Input: part model. Units: mm. Frame: model coordinates. A direction names the side the tool comes from. Give positions to 0.01 mm unless a question says otherwise; leave off trailing zeros. Loops run counter-clockwise (first coordinate to the right, second up) from the corner with the lowest first, then second, coordinate; pieces in that order, holes last. Notation, with made-up numbers: (68.5, 16.25) - (108.5, 16.25) arc R11 cw to (108.5, 30.25) - close; hole circle Ø11 at (58, 25). An arc over 180 degrees is marked (long way). Answer as a JSON object with one key per item and string values. Group by question number.
(1) Pin query (flat end, axial travel): P1, Ø4, axis at x = -78.5, y = 43.5, coming from the -Z side; P2, Ø10, axis at x = -23.5, y = 35, coming from the -Z side; P3, Ø6, axis at x = -40.5, y = 5, coming from the -Z side. Return the tip coordinate at first contact, or that it passes through.
(2) Mould query, pull axis X, two halves, no side actions, for faces 4 (the flat face through (-78, 43, -15.147)), 5 (the flat face through (-80, 3, 1)), 6 (the flat face through (80, 3, 1)), 7 (the flat face through (75, -4, 6)). Classes: +X half, -X half, draft (parallel to the pull), parting line (faces both ways), or undercut.
(3) Access query for faces 1 (the flat face through (77, 43, -15.147)), 2 (the flat face through (-1, -35, 6)), 3 (the flat face through (1, 37, -15.147)). Directions: +Z, -Z, +X, -X, +Y, -Y. A direction counts if a zero-diameter tool reaches every point of the face in a straight line with its end or side. Return the directions, or none.
(4) Section query C-C (y = -12.5). Return loops of the section in (x, z), plus the area to 3 significant figures.
(5) Section query A-A (z = -2). Return loops of the section in (x, y), plus the area to 3 significant figures.
(6) Section query D-D (x = 22). Return loops of the section in (y, z), plus the area to 3 significant figures.
(7) Material intervals for L1, parallel to X at y = 15, z = -1.5; L2, parallel to Y at x = 52, z = 79.5; L3, parallel to Y at x = 17.5, z = -56, sorted ascending.
(8) Section query B-B (z = -60). Return loops of the section in (x, y), plus the area to 3 significant figures.
```python
from build123d import *

# Parameters (mm, degrees)
SKETCH1_W           = 200
SKETCH1_H           = 80
BOSS_EXTRUDE1_DEPTH = 80
SKETCH2_W           = 150
SKETCH2_H           = 70
CUT_EXTRUDE2_DEPTH  = 190
FILLET5_R           = 85
CUT_EXTRUDE6_DEPTH  = 10
SKETCH9_W           = 5
SKETCH9_H           = 115.147186258
BOSS_EXTRUDE2_DEPTH = 7
SKETCH10_W          = 5
SKETCH10_H          = 115.147186258
BOSS_EXTRUDE3_DEPTH = 7
SKETCH13_W          = 100
SKETCH13_H          = 3.5
CUT_EXTRUDE9_DEPTH  = 1
SKETCH14_W          = 100
SKETCH14_H          = 3.5
CUT_EXTRUDE10_DEPTH = 1


with BuildPart() as part:
    # Sketch1 → Boss-Extrude1 (new, symmetric)
    with BuildSketch(Plane(origin=(0, 0, 0), x_dir=(0, 0, -1), z_dir=(1, 0, 0))):
        Rectangle(SKETCH1_W, SKETCH1_H)
    extrude(amount=BOSS_EXTRUDE1_DEPTH, both=True)

    # Sketch2 → Cut-Extrude2 (cut)
    with BuildSketch(Plane.XY.offset(100)):
        Rectangle(SKETCH2_W, SKETCH2_H)
    extrude(amount=-CUT_EXTRUDE2_DEPTH, mode=Mode.SUBTRACT)

    # Fillet5
    # the kernel refuses this fillet: 85 mm, written as the material it adds along each edge
    with BuildSketch(Plane(origin=(-75, 35, -90), x_dir=(0, 0, 1), z_dir=(1, 0, 0))) as fillet5_piece_1:
        with BuildLine():
            CenterArc((83.666002653, 85), FILLET5_R, 190.164248622, 79.835751378)
            Line((0, 70), (-1.673320053, 69.7))
            ThreePointArc((-1.673320053, 69.7), (-1.7, 35), (-1.7, 0))
            Line((-1.7, 0), (0, -1.7))
            Line((0, -1.7), (83.666002653, -1.7))
            Line((83.666002653, -1.7), (83.666002653, 0))
        make_face()
    extrude(amount=150)
    # the kernel refuses this fillet: 85 mm, written as the material it takes off along each edge
    with BuildSketch(Plane(origin=(-292.132034356, 40, -100), x_dir=(0, -1, 0), z_dir=(1, 0, 0))) as fillet5_2_piece_1:
        with BuildLine():
            CenterArc((85, -84.852813742), FILLET5_R, 93.372286683, 86.627713317)
            Line((0, -84.852813742), (-1.7, -84.852813742))
            Line((-1.7, -84.852813742), (-1.7, 0))
            Line((-1.7, 0), (0, 1.7))
            ThreePointArc((0, 1.7), (40, 1.7), (79.9, 1.697056275))
            Line((79.9, 1.697056275), (80, 0))
        make_face()
    extrude(amount=584.264068712, mode=Mode.SUBTRACT)

    # Sketch8 → Cut-Extrude6 (cut)
    with BuildSketch(Plane(origin=(0, 40, 0), x_dir=(1, 0, 0), z_dir=(0, 1, 0))):
        Polygon((0, 15.147186258), (-75, 15.147186258), (-75, -100), (75, -100), (75, 15.147186258), align=None)
    extrude(amount=-CUT_EXTRUDE6_DEPTH, mode=Mode.SUBTRACT)

    # Sketch9 → Boss-Extrude2 (add)
    with BuildSketch(Plane(origin=(0, 40, 0), x_dir=(1, 0, 0), z_dir=(0, 1, 0))):
        with Locations((-77.5, -42.426406871)):
            Rectangle(SKETCH9_W, SKETCH9_H)
    extrude(amount=BOSS_EXTRUDE2_DEPTH)

    # Sketch10 → Boss-Extrude3 (add)
    with BuildSketch(Plane(origin=(0, 40, 0), x_dir=(1, 0, 0), z_dir=(0, 1, 0))):
        with Locations((77.5, -42.426406871)):
            Rectangle(SKETCH10_W, SKETCH10_H)
    extrude(amount=BOSS_EXTRUDE3_DEPTH)

    # Sketch13 → Cut-Extrude9 (cut)
    with BuildSketch(Plane(origin=(-75, 0, 0), x_dir=(0, 0, -1), z_dir=(1, 0, 0))):
        with Locations((-34.852813742, 41.75)):
            Rectangle(SKETCH13_W, SKETCH13_H)
    extrude(amount=-CUT_EXTRUDE9_DEPTH, mode=Mode.SUBTRACT)

    # Sketch14 → Cut-Extrude10 (cut)
    with BuildSketch(Plane.ZY.offset(-75)):
        with Locations((34.852813742, 41.75)):
            Rectangle(SKETCH14_W, SKETCH14_H)
    extrude(amount=-CUT_EXTRUDE10_DEPTH, mode=Mode.SUBTRACT)


solid = part.part
```
Recorded:
{
 "1": {"P1": "stops at z = -15.15", "P2": "stops at z = -55.15", "P3": "stops at z = -85.97"},
 "2": {"face 4": "draft", "face 5": "-X half", "face 6": "+X half", "face 7": "undercut"},
 "3": {"face 1": "-Z, +X, -X, +Y", "face 2": "+Z", "face 3": "+Z, +Y"},
 "4": {"outline": "(-80, -93.69) - (80, -93.69) - (80, 100) - (75, 100) - (75, -82.61) - (-75, -82.61) - (-75, 100) - (-80, 100) - close", "area": "3,600 mm^2"},
 "5": {"outline": "(-80, -40) - (80, -40) - (80, 47) - (75, 47) - (75, 43.5) - (76, 43.5) - (76, 40) - (75, 40) - (75, -35) - (-75, -35) - (-75, 40) - (-76, 40) - (-76, 43.5) - (-75, 43.5) - (-75, 47) - (-80, 47) - close", "area": "1,610 mm^2"},
 "6": {"outline": "(-40, -100) arc R85 ccw to (40, -15.15) - (34.54, -15.15) arc R85 cw to (-35, -90) - (-35, 100) - (-40, 100) - close", "area": "2,030 mm^2"},
 "7": {"L1": "x = -80 to -75, 75 to 80", "L2": "y = -40 to -35", "L3": "y = -40 to -35, 18.98 to 29.54"},
 "8": {"outline": "(-80, -40) - (80, -40) - (80, 27.2) - (-80, 27.2) - close; hole (-75, -35) - (75, -35) - (75, 15.92) - (-75, 15.92) - close", "area": "3,110 mm^2"}
}
